from build123d import *

# Parameters (mm, degrees)
PAD001_DEPTH    = 98
SKETCH001_R     = 2.6
SKETCH001_R_2   = 8
POCKET_DEPTH    = 8
SKETCH002_R     = 9
SKETCH002_R_2   = 2.5
POCKET001_DEPTH = 10


with BuildPart() as part:
    # Sketch → Pad001 (new body)
    with BuildSketch(Plane.XY):
        with BuildLine():
            Line((6.35, 10.35), (6.35, 67))
            Line((6.35, 67), (0, 67))
            Line((0, 67), (0, 0))
            Line((0, 0), (51.8, 0))
            Line((51.8, 0), (51.8, 6.35))
            Line((51.8, 6.35), (10.35, 6.35))
            ThreePointArc((6.35, 10.35), (7.521573, 7.521573), (10.35, 6.35))
        make_face()
    extrude(amount=PAD001_DEPTH)

    # Sketch001 → Pocket (cut)
    with BuildSketch(Plane(origin=(0, 0, 0), x_dir=(0, -1, 0), z_dir=(-1, 0, 0))):
        with Locations((-60, 88)):
            Circle(SKETCH001_R)
        with Locations((-20, 78)):
            Circle(SKETCH001_R)
        with Locations((-30, 53)):
            Circle(SKETCH001_R_2)
        with Locations((-15, 34)):
            Circle(SKETCH001_R_2)
        with BuildLine():
            Line((-68, 0), (-68, 42))
            Line((-68, 42), (-56.999999, 42))
            ThreePointArc((-57.000001, 26), (-49, 33.999999), (-56.999999, 42))
            Line((-67, 26), (-57.000001, 26))
            Line((-67, 26), (-67, 7.999993))
            ThreePointArc((-67, 7.999993), (-64.656849, 2.343141), (-58.999993, 0))
            Line((-68, 0), (-58.999993, 0))
        make_face()
    extrude(amount=-POCKET_DEPTH, mode=Mode.SUBTRACT)

    # Sketch002 → Pocket001 (cut)
    with BuildSketch(Plane.XZ):
        with Locations((29, 26.5)):
            Circle(SKETCH002_R)
        with Locations((15.564971, 39.935029)):
            Circle(SKETCH002_R_2)
        with Locations((29, 45.5)):
            Circle(SKETCH002_R_2)
        with Locations((42.435029, 39.935029)):
            Circle(SKETCH002_R_2)
        with Locations((15.564971, 13.064971)):
            Circle(SKETCH002_R_2)
        with Locations((29, 7.5)):
            Circle(SKETCH002_R_2)
        with Locations((42.435029, 13.064971)):
            Circle(SKETCH002_R_2)
        with BuildLine():
            Line((6.35, 61.000036), (6.35, 98))
            Line((6.35, 98), (51.8, 98))
            Line((51.8, 98), (51.8, 45))
            ThreePointArc((51.8, 45), (49.456854, 50.656854), (43.8, 53))
            Line((43.8, 53), (14.35, 53))
            ThreePointArc((14.35, 53), (8.693133, 55.343159), (6.35, 61.000036))
        make_face()
        with BuildLine():
            ThreePointArc((43.8, 0), (49.456854, 2.343146), (51.8, 8))
            Line((51.8, 8), (51.8, 0))
            Line((51.8, 0), (43.8, 0))
        make_face()
    extrude(amount=-POCKET001_DEPTH, mode=Mode.SUBTRACT)


solid = part.part
Can you work these out from the model? Positions are in its coordinate system, mm. A direction names the side the tool comes from. Round coordinates to 2 decimals unless told otherwise and drop trailing zeros. Write each loop counter-clockwise with the first axis right and the second up, starting at its lowest first coordinate (ties: lowest second). Pieces come first, ordered by that corner, then holes. Notation, with made-up numbers: M 38,64 L 54,64 A19 ccw 54,68 Z; hole C 40.25,87.5 d4. An arc over 180 degrees is marked long. Use CSV: the item, a comma, the result in double quotes.
(1) Imagine slicing it at D-D (x = 35). Write out the boundary of the cut face in (y, z), plus the area to 3 significant figures.
Check values:
outline,"M 0,0 L 6.35,0 L 6.35,19.79 L 0,19.79 Z; M 0,33.21 L 6.35,33.21 L 6.35,53 L 0,53 Z"
area,"251 mm^2"
(2) I need wall thicknesses on line 1 along Z through (x, y) = (3.75, 60); line 2 along Y through (x, z) = (12, 30). Which ranges of each line are inside material? Lowest first, please.
Check values:
line 1,"0.06 to 26, 42 to 85.4, 90.6 to 98"
line 2,"0 to 6.35"
(3) We'd pull the mould along Y, two halves only. Please class faces 1 (the cylindrical face through (3.1, 35.9, 58.4)), 2 (the flat face through (6, 19, 0)), 3 (the flat face through (19.8, 0, 26.5)), 4 (the cylindrical face through (3.131, 64.719, 2.406)): +Y half, -Y half, draft (parallel to the pull), parting line (faces both ways), or undercut.
Check values:
face 1,"undercut"
face 2,"draft"
face 3,"-Y half"
face 4,"+Y half"
(4) Imagine slicing it at C-C (y = 15). Write out the boundary of the cut face in (x, z).
Check values:
outline,"M 0,0 L 6.35,0 L 6.35,26 L 0,26 Z; M 0,42 L 6.35,42 L 6.35,98 L 0,98 Z"
(5) On a 3-axis mill with a long thin cutter (end or side, diameter ignored), from which of +Z, -Z, +X, -X, +Y, -Y can I reach the whole of each face in a straight line? I mean faces 5 (the cylindrical face through (27, 3, 6)), 6 (the flat face through (29, 3, 53)), 7 (the flat face through (36, 6.35, 20.6)), 8 (the flat face through (3, 62, 26)). Say none if no direction works.
Check values:
face 5,"+Y, -Y"
face 6,"+Z, +X, +Y, -Y"
face 7,"+Z, -Z, +X, +Y"
face 8,"+X, -X, +Y"
(6) Imagine slicing it at A-A (x = 29). Write out the boundary of the cut face in (y, z).
Check values:
outline,"M 0,0 L 6.35,0 L 6.35,5 L 0,5 Z; M 0,10 L 6.35,10 L 6.35,17.5 L 0,17.5 Z; M 0,35.5 L 6.35,35.5 L 6.35,43 L 0,43 Z; M 0,48 L 6.35,48 L 6.35,53 L 0,53 Z"
(7) I'm going to push flat-ended pins straight in: pin 1 (6.5 mm diameter, centred on x = 29, z = 45.5, fed in from +Y); pin 2 (8.5 mm diameter, centred on y = 20, z = 78, fed in from +X); pin 3 (3 mm diameter, centred on x = 24.5, y = 2, fed in from +Z). Where does each tip first touch, or does it pass through?
Check values:
pin 1,"y = 6.35"
pin 2,"x = 6.35"
pin 3,"z = 53"
